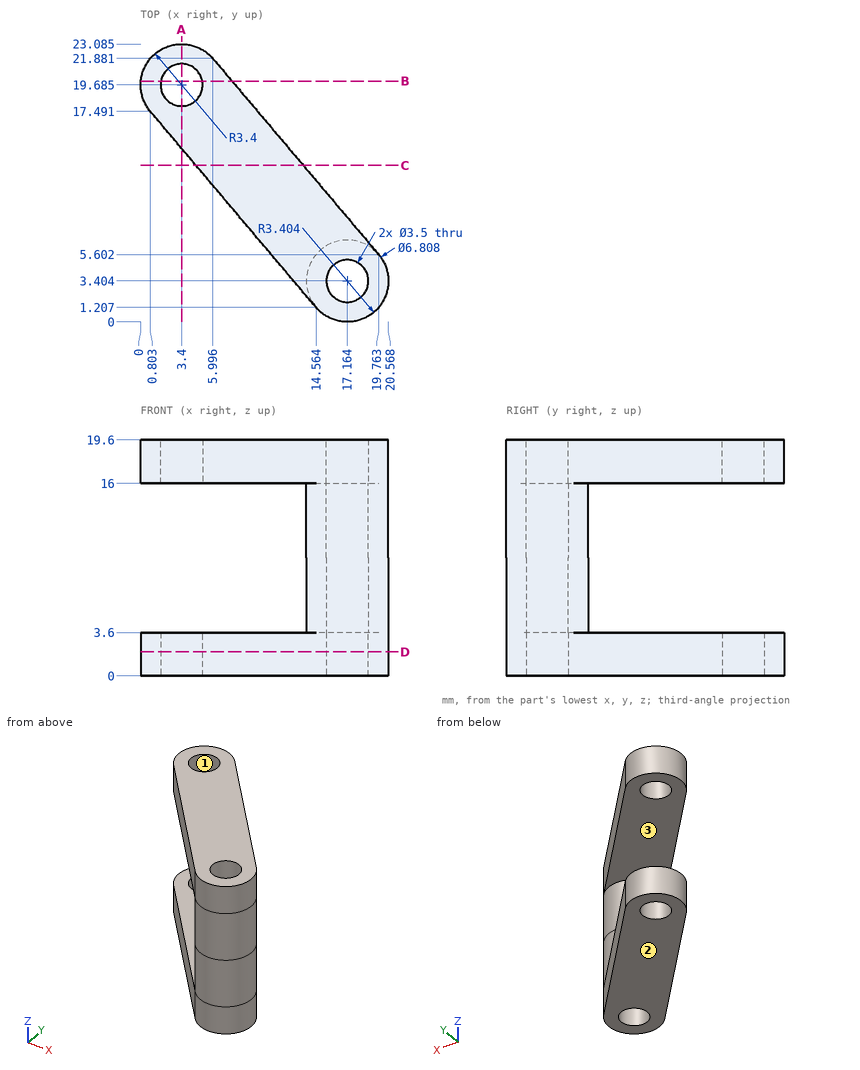
The drawing under review shows one solid part. Ordinate dimensions are in mm from its lowest x, y, z. Coordinates: 2 decimals unless noted, no trailing zeros. Order: outer loops, then holes, each group sorted by start corner. A loop starts at its lowest first (then second) coordinate and runs counter-clockwise, first axis right, second up. Notation, with made-up numbers: (49.25, 5) -> (82.25, 5) arc R15 cw to (82.25, 24) -> close; hole circle Ø4 at (85, 24.25). An arc over 180 degrees is marked (long way). Answer as CSV lines item,"result".
Q1. Clearance check with flat-ended pins moving along their axes: pin 1 Ø5 at (x, z) = (14.5, 4) entering from +Y (1 decimal); pin 2 Ø2 at (x, z) = (2, 15.5) entering from -Y. State where each tip first meets the part, or that it passes through.
Model answer:
pin 1,"stops at y = 14.7"
pin 2,"stops at y = 15.05"
Q2. We need section D-D (z = 2). Count the separate pieces of the cut face and the enclosed holes in it, plus the area to 3 significant figures.
Model answer:
separate pieces,"1"
enclosed holes,"2"
area,"162 mm2"
Q3. We need section C-C (y = 13). State the section outline as (x, z) points.
Model answer:
outline,"(4.6, 0) -> (13.51, 0) -> (13.51, 3.6) -> (4.6, 3.6) -> close; (4.6, 16) -> (13.51, 16) -> (13.51, 19.6) -> (4.6, 19.6) -> close"
Q4. We need section B-B (y = 20). State the section outline as (x, z) points (1 decimal).
Model answer:
outline,"(0, 0) -> (1.7, 0) -> (1.7, 3.6) -> (0, 3.6) -> close; (0, 16) -> (1.7, 16) -> (1.7, 19.6) -> (0, 19.6) -> close; (5.1, 0) -> (7.6, 0) -> (7.6, 3.6) -> (5.1, 3.6) -> close; (5.1, 16) -> (7.6, 16) -> (7.6, 19.6) -> (5.1, 19.6) -> close"
Q5. We need section A-A (x = 3.4). State the section outline as (y, z) points (1 decimal).
Model answer:
outline,"(14.4, 0) -> (17.9, 0) -> (17.9, 3.6) -> (14.4, 3.6) -> close; (14.4, 16) -> (17.9, 16) -> (17.9, 19.6) -> (14.4, 19.6) -> close; (21.4, 0) -> (23.1, 0) -> (23.1, 3.6) -> (21.4, 3.6) -> close; (21.4, 16) -> (23.1, 16) -> (23.1, 19.6) -> (21.4, 19.6) -> close"
Q6. Draft analysis for pull direction Z (two halves, no side actions). For the marked faces 1, 2 and 3, state which applies: released by +Z, released by -Z, zero draft, split by the parting line, or undercut.
Model answer:
face 1,"zero draft"
face 2,"released by -Z"
face 3,"undercut"
Q7. Wall thickness on line 1 along Z through (x, y) = (11.25, 6.5); line 2 along Y through (x, z) = (18.25, 18.5) (1 decimal); line 3 along Y through (x, z) = (16.25, 6) (1 decimal): over which ranges is each line inside the solid? List them lowest first. Write a range as [from, to].
Model answer:
line 1,"z = [0, 3.6], [16, 19.6]"
line 2,"y = [0.2, 2], [4.8, 7.4]"
line 3,"y = [0.1, 1.9], [4.9, 6.7]"
